The model under review builds one solid part; all positions refer to its coordinate system, in mm. A direction names the side the tool comes from. Give positions to 0.01 mm unless a question says otherwise; leave off trailing zeros. Order: outer loops, then holes, each group sorted by start corner. A loop starts at its lowest first (then second) coordinate and runs counter-clockwise, first axis right, second up. Notation, with made-up numbers: (19, 89.25) - (70, 89.25) arc R17 ccw to (70, 100.25) - close; hole circle Ø5 at (20.5, 48). An arc over 180 degrees is marked (long way). Use CSV: the item, a comma, the result in double quotes.
```python
from build123d import *

# Parameters (mm, degrees)
SKETCH_1_W          = 57
SKETCH_1_H          = 51
SKETCH_1_W_2        = 3.4
SKETCH_1_H_2        = 3.4
SKETCH_1_W_3        = 7
SKETCH_1_H_3        = 42
EXTRUDE_1_DEPTH     = 3
SKETCH_2_W          = 31
SKETCH_2_H          = 47
CUT_EXTRUDE_1_DEPTH = 1
SKETCH_3_R          = 1.25
CUT_EXTRUDE_2_DEPTH = 42.060930335
SKETCH_5_W          = 57
SKETCH_5_H          = 3
EXTRUDE_2_DEPTH     = 1
SKETCH_6_W          = 57
SKETCH_6_H          = 3
EXTRUDE_3_DEPTH     = 1
SKETCH_7_W          = 10
SKETCH_7_H          = 3
EXTRUDE_4_DEPTH     = 6
SKETCH_8_W          = 31
SKETCH_8_H          = 3
EXTRUDE_5_DEPTH     = 6
CUT_EXTRUDE_3_REACH = 63.082
SKETCH_9_R          = 1.15
CUT_EXTRUDE_4_REACH = 63.082
SKETCH_10_R         = 1.15
SKETCH_12_W         = 57
SKETCH_12_H         = 53
SKETCH_12_R         = 1.25
SKETCH_12_W_2       = 3.4
SKETCH_12_H_2       = 3.4
SKETCH_12_W_3       = 7
SKETCH_12_H_3       = 42
EXTRUDE_6_DEPTH     = 0.5
EXTRUDE_START       = 0.2
SKETCH_13_R         = 1.15
EXTRUDE_7_DEPTH     = 0.2
SKETCH_14_R         = 1.15
EXTRUDE_8_DEPTH     = 0.2
SKETCH_15_R         = 1.15
CUT_EXTRUDE_5_DEPTH = 0.2
CUT_EXTRUDE_START   = -0.2
SKETCH_16_R         = 1.15
CUT_EXTRUDE_6_DEPTH = 0.2


with BuildPart() as part:
    # 草图1 → 凸台-拉伸1 (new body)
    with BuildSketch(Plane.XY):
        with Locations((0.5, 3.5)):
            Rectangle(SKETCH_1_W, SKETCH_1_H)
        with Locations((13.3, 0.3)):
            Rectangle(SKETCH_1_W_2, SKETCH_1_H_2, mode=Mode.SUBTRACT)
        with Locations((21.5, 3.5)):
            Rectangle(SKETCH_1_W_3, SKETCH_1_H_3, mode=Mode.SUBTRACT)
        with Locations((-20.5, 3.5)):
            Rectangle(SKETCH_1_W_3, SKETCH_1_H_3, mode=Mode.SUBTRACT)
    extrude(amount=EXTRUDE_1_DEPTH)

    # 草图2 → 切除-拉伸1 (cut)
    with BuildSketch(Plane.XY.offset(3)):
        with Locations((0.5, 3.5)):
            Rectangle(SKETCH_2_W, SKETCH_2_H)
    extrude(amount=-CUT_EXTRUDE_1_DEPTH, mode=Mode.SUBTRACT)

    # 草图3 → 切除-拉伸2 (cut, through all)
    with BuildSketch(Plane.XY.offset(2)):
        with Locations((-12.2, 18.3)):
            Circle(SKETCH_3_R)
        with Locations((13.2, 18.1)):
            Circle(SKETCH_3_R)
        with Locations((12.9, -17.3)):
            Circle(SKETCH_3_R)
        with Locations((-11.9, -17.3)):
            Circle(SKETCH_3_R)
    extrude(amount=-CUT_EXTRUDE_2_DEPTH, mode=Mode.SUBTRACT)

    # 草图5 → 凸台-拉伸2 (add)
    with BuildSketch(Plane(origin=(0, 29, 0), x_dir=(1, 0, 0), z_dir=(0, 1, 0))):
        with Locations((0.5, -1.5)):
            Rectangle(SKETCH_5_W, SKETCH_5_H)
    extrude(amount=EXTRUDE_2_DEPTH)

    # 草图6 → 凸台-拉伸3 (add)
    with BuildSketch(Plane(origin=(0, -22, 0), x_dir=(-1, 0, 0), z_dir=(0, -1, 0))):
        with Locations((-0.5, -1.5)):
            Rectangle(SKETCH_6_W, SKETCH_6_H)
    extrude(amount=EXTRUDE_3_DEPTH)

    # 草图7 → 凸台-拉伸4 (add)
    with BuildSketch(Plane.XY.offset(3)):
        with Locations((-10, -21.5)):
            Rectangle(SKETCH_7_W, SKETCH_7_H)
        with Locations((11, -21.5)):
            Rectangle(SKETCH_7_W, SKETCH_7_H)
    extrude(amount=EXTRUDE_4_DEPTH)

    # 草图8 → 凸台-拉伸5 (add)
    with BuildSketch(Plane.XY.offset(3)):
        with Locations((0.5, 28.5)):
            Rectangle(SKETCH_8_W, SKETCH_8_H)
    extrude(amount=EXTRUDE_5_DEPTH)

    # 草图9 → 切除-拉伸3 (cut, up to next)
    with BuildSketch(Plane.XZ.offset(23), mode=Mode.PRIVATE) as cut_extrude_3_sk1:
        with Locations(Location((-10, 7, 0), (0, 0, 270))):
            Circle(SKETCH_9_R)
    cut_extrude_3_tool1 = extrude(cut_extrude_3_sk1.sketch, amount=-CUT_EXTRUDE_3_REACH, mode=Mode.PRIVATE) & part.part
    # 草图9 → 切除-拉伸3 (cut, up to next)
    with BuildSketch(Plane.XZ.offset(23), mode=Mode.PRIVATE) as cut_extrude_3_sk2:
        with Locations(Location((11, 7, 0), (0, 0, 270))):
            Circle(SKETCH_9_R)
    cut_extrude_3_tool2 = extrude(cut_extrude_3_sk2.sketch, amount=-CUT_EXTRUDE_3_REACH, mode=Mode.PRIVATE) & part.part
    add(cut_extrude_3_tool1.solids().sort_by_distance((-10, -23, 7))[0], mode=Mode.SUBTRACT)
    add(cut_extrude_3_tool2.solids().sort_by_distance((11, -23, 7))[0], mode=Mode.SUBTRACT)

    # 草图10 → 切除-拉伸4 (cut, up to next)
    with BuildSketch(Plane(origin=(0, 30, 0), x_dir=(1, 0, 0), z_dir=(0, 1, 0)), mode=Mode.PRIVATE) as cut_extrude_4_sk1:
        with Locations(Location((-10, -7, 0), (0, 0, 90))):
            Circle(SKETCH_10_R)
    cut_extrude_4_tool1 = extrude(cut_extrude_4_sk1.sketch, amount=-CUT_EXTRUDE_4_REACH, mode=Mode.PRIVATE) & part.part
    # 草图10 → 切除-拉伸4 (cut, up to next)
    with BuildSketch(Plane(origin=(0, 30, 0), x_dir=(1, 0, 0), z_dir=(0, 1, 0)), mode=Mode.PRIVATE) as cut_extrude_4_sk2:
        with Locations(Location((0.5, -7, 0), (0, 0, 270))):
            Circle(SKETCH_10_R)
    cut_extrude_4_tool2 = extrude(cut_extrude_4_sk2.sketch, amount=-CUT_EXTRUDE_4_REACH, mode=Mode.PRIVATE) & part.part
    # 草图10 → 切除-拉伸4 (cut, up to next)
    with BuildSketch(Plane(origin=(0, 30, 0), x_dir=(1, 0, 0), z_dir=(0, 1, 0)), mode=Mode.PRIVATE) as cut_extrude_4_sk3:
        with Locations(Location((11, -7, 0), (0, 0, 90))):
            Circle(SKETCH_10_R)
    cut_extrude_4_tool3 = extrude(cut_extrude_4_sk3.sketch, amount=-CUT_EXTRUDE_4_REACH, mode=Mode.PRIVATE) & part.part
    add(cut_extrude_4_tool1.solids().sort_by_distance((-10, 30, 7))[0], mode=Mode.SUBTRACT)
    add(cut_extrude_4_tool2.solids().sort_by_distance((0.5, 30, 7))[0], mode=Mode.SUBTRACT)
    add(cut_extrude_4_tool3.solids().sort_by_distance((11, 30, 7))[0], mode=Mode.SUBTRACT)

    # 草图12 → 凸台-拉伸6 (add)
    with BuildSketch(Plane(origin=(0, 0, 0), x_dir=(-1, 0, 0), z_dir=(0, 0, -1))):
        with Locations((-0.5, 3.5)):
            Rectangle(SKETCH_12_W, SKETCH_12_H)
        with Locations(Location((-12.9, -17.3, 0), (0, 0, 180))):
            Circle(SKETCH_12_R, mode=Mode.SUBTRACT)
        with Locations(Location((12.2, 18.3, 0), (0, 0, 180))):
            Circle(SKETCH_12_R, mode=Mode.SUBTRACT)
        with Locations(Location((-13.2, 18.1, 0), (0, 0, 180))):
            Circle(SKETCH_12_R, mode=Mode.SUBTRACT)
        with Locations(Location((11.9, -17.3, 0), (0, 0, 180))):
            Circle(SKETCH_12_R, mode=Mode.SUBTRACT)
        with Locations((-13.3, 0.3)):
            Rectangle(SKETCH_12_W_2, SKETCH_12_H_2, mode=Mode.SUBTRACT)
        with Locations((20.5, 3.5)):
            Rectangle(SKETCH_12_W_3, SKETCH_12_H_3, mode=Mode.SUBTRACT)
        with Locations((-21.5, 3.5)):
            Rectangle(SKETCH_12_W_3, SKETCH_12_H_3, mode=Mode.SUBTRACT)
    extrude(amount=EXTRUDE_6_DEPTH)

    # 草图13 → 凸台-拉伸7 (add)
    with BuildSketch(Plane(origin=(0, 30, 0), x_dir=(1, 0, 0), z_dir=(0, 1, 0)).offset(EXTRUDE_START)):
        Polygon((16, -3), (29, -3), (29, 0.5), (-28, 0.5), (-28, -3), (-15, -3), (-15, -9), (16, -9), align=None)
        with Locations(Location((0.5, -7, 0), (0, 0, 270))):
            Circle(SKETCH_13_R, mode=Mode.SUBTRACT)
        with Locations(Location((11, -7, 0), (0, 0, 90))):
            Circle(SKETCH_13_R, mode=Mode.SUBTRACT)
        with Locations(Location((-10, -7, 0), (0, 0, 90))):
            Circle(SKETCH_13_R, mode=Mode.SUBTRACT)
    extrude(amount=-EXTRUDE_7_DEPTH)

    # 草图14 → 凸台-拉伸8 (add)
    with BuildSketch(Plane(origin=(0, -23, 0), x_dir=(-1, 0, 0), z_dir=(0, -1, 0))):
        Polygon((-29, 0.5), (-29, -3), (-16, -3), (-16, -9), (-6, -9), (-6, -3), (5, -3), (5, -9), (15, -9), (15, -3), (28, -3), (28, 0.5), align=None)
        with Locations(Location((-11, -7, 0), (0, 0, 90))):
            Circle(SKETCH_14_R, mode=Mode.SUBTRACT)
        with Locations(Location((10, -7, 0), (0, 0, 90))):
            Circle(SKETCH_14_R, mode=Mode.SUBTRACT)
    extrude(amount=EXTRUDE_8_DEPTH)

    # 草图15 → 切除-拉伸5 (cut)
    with BuildSketch(Plane(origin=(0, -20, 0), x_dir=(1, 0, 0), z_dir=(0, 1, 0))):
        Polygon((16, -2), (-15, -2), (-15, -3), (-15, -9), (-5, -9), (-5, -3), (6, -3), (6, -9), (16, -9), (16, -3), align=None)
        with Locations(Location((11, -7, 0), (0, 0, 90))):
            Circle(SKETCH_15_R, mode=Mode.SUBTRACT)
        with Locations(Location((-10, -7, 0), (0, 0, 90))):
            Circle(SKETCH_15_R, mode=Mode.SUBTRACT)
    extrude(amount=-CUT_EXTRUDE_5_DEPTH, mode=Mode.SUBTRACT)

    # 草图16 → 切除-拉伸6 (cut)
    with BuildSketch(Plane.XZ.offset(-27).offset(CUT_EXTRUDE_START)):
        Polygon((-15, 2), (16, 2), (16, 3), (16, 9), (-15, 9), (-15, 3), align=None)
        with Locations(Location((0.5, 7, 0), (0, 0, 90))):
            Circle(SKETCH_16_R, mode=Mode.SUBTRACT)
        with Locations(Location((11, 7, 0), (0, 0, 90))):
            Circle(SKETCH_16_R, mode=Mode.SUBTRACT)
        with Locations(Location((-10, 7, 0), (0, 0, 90))):
            Circle(SKETCH_16_R, mode=Mode.SUBTRACT)
    extrude(amount=CUT_EXTRUDE_6_DEPTH, mode=Mode.SUBTRACT)


solid = part.part
```
Item 1: Take a section at A-A, the plane z = 7. State how many separate pieces and enclosed holes the cut face has, and give its area (4 significant figures).
Results list:
separate pieces,"8"
enclosed holes,"0"
area,"118.5 mm2"
Item 2: Tool access review of faces 1 (the face through (-15, -22, 6)), 2 (the face through (0, 4, 2)), 3 (the face through (16, -22, 6)), 4 (the face through (-5, -22, 6)), 5 (the face through (11.6, 0, 1)): name each direction out of +Z, -Z, +X, -X, +Y, -Y from which nothing blocks a thin tool from reaching the whole face with its end or side.
Results list:
face 1,"+Z, -X, +Y, -Y"
face 2,"+Z"
face 3,"+Z, +X, +Y, -Y"
face 4,"+Z, -Y"
face 5,"+Z, -Z"
Item 3: Wall thickness on L1, parallel to X at y = 29.1, z = 7; L2, parallel to Y at x = -12, z = 0.25; L3, parallel to X at y = -17.3, z = 0.2: over which ranges is each line inside the solid? List them lowest first.
Results list:
L1,"x = -15 to -11.15, -8.85 to -0.65, 1.65 to 9.85, 12.15 to 16"
L2,"y = -23.2 to -18.55, -16.05 to 17.07, 19.53 to 30.2"
L3,"x = -28 to -24, -17 to -13.15, -10.65 to 11.65, 14.15 to 18, 25 to 29"
Item 4: Take a section at B-B, the plane y = -8. Give the boundary of the cut face in (x, z), and give its area (4 significant figures).
Results list:
outline,"(-28, -0.5) - (-24, -0.5) - (-24, 3) - (-28, 3) - close; (-17, -0.5) - (18, -0.5) - (18, 3) - (16, 3) - (16, 2) - (-15, 2) - (-15, 3) - (-17, 3) - close; (25, -0.5) - (29, -0.5) - (29, 3) - (25, 3) - close"
area,"119.5 mm2"
Item 5: Take a section at C-C, the plane x = 21. Give the boundary of the cut face in (y, z), and give its area (3 significant figures).
Results list:
outline,"(-23.2, -0.5) - (-17.5, -0.5) - (-17.5, 3) - (-23.2, 3) - close; (24.5, -0.5) - (30.2, -0.5) - (30.2, 3) - (24.5, 3) - close"
area,"39.9 mm2"
Item 6: Clearance check with flat-ended pins moving along their axes: pin 1 (2.5 mm diameter, centred on y = 29, z = 5, fed in from +X); pin 2 (8 mm diameter, centred on x = -18.5, y = 9, fed in from +Z); pin 3 (3.5 mm diameter, centred on y = -21.5, z = 7, fed in from -X). State where each tip first meets the part, or that it passes through.
Results list:
pin 1,"stops at x = 16"
pin 2,"stops at z = 3"
pin 3,"stops at x = -15"
Item 7: Mouldability with a two-part tool opening along Y and no side actions: class faces 6 (the face through (13, 2, 1)), 7 (the face through (18, 3, 1)), 8 (the face through (11, -22, 9)) as pulls with the +Y half, pulls with the -Y half, needs draft (parallel to the pull), parting line crosses it, or undercut.
Results list:
face 6,"undercut"
face 7,"undercut"
face 8,"needs draft"
Item 8: Take a section at D-D, the plane x = 12.9. Give the boundary of the cut face in (y, z).
Results list:
outline,"(-23.2, -0.5) - (-18.55, -0.5) - (-18.55, 2) - (-20.2, 2) - (-20.2, 9) - (-23.2, 9) - close; (-16.05, -0.5) - (-1.4, -0.5) - (-1.4, 2) - (-16.05, 2) - close; (2, -0.5) - (16.89, -0.5) - (16.89, 2) - (2, 2) - close; (19.31, -0.5) - (30.2, -0.5) - (30.2, 9) - (27.2, 9) - (27.2, 2) - (19.31, 2) - close"
